Study the drawing (mm; zero at the part's minimum x, y, z) and answer. A direction names the side the tool comes from. Coordinates: 2 decimals unless noted, no trailing zeros. Loops run counter-clockwise (first coordinate to the right, second up) from the corner with the lowest first, then second, coordinate; pieces in that order, holes last. Notation, with made-up numbers: (86, 57.25) - (118, 57.25) arc R28 cw to (118, 91.25) - close; hole circle Ø1 at (45, 24). An arc over 180 degrees is marked (long way). Use one line per item in the form item = value.
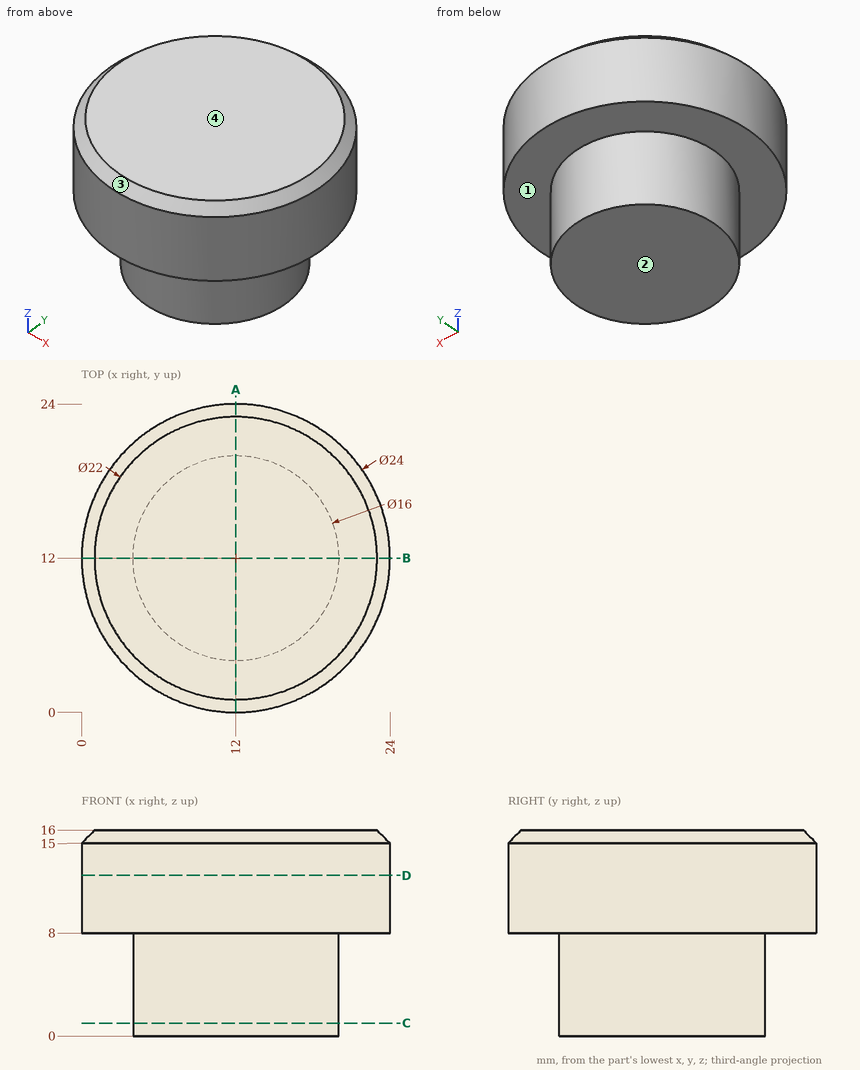
Item 1: The part is cut by section C-C on z = 1. Give the vertices of the cut face in (x, y).
Results below:
outline = circle Ø16 at (12, 12)
Item 2: For a pull along X with two mould halves and no side action, classify the marked faces 3 and 4 as +X half, -X half, draft (parallel to the pull), parting line (faces both ways), or undercut.
Results below:
face_3 = parting line
face_4 = draft
Item 3: The part is cut by section D-D on z = 12.5. Give the vertices of the cut face in (x, y), plus the area to 3 significant figures.
Results below:
outline = circle Ø24 at (12, 12)
area = 452 mm²
Item 4: Each of these flat-tipped pins is pushed along its axis until it touches: P1, Ø2, axis at x = 21, y = 16, coming from the -Z side; P2, Ø1.5, axis at y = 3.5, z = 14, coming from the -X side; P3, Ø2, axis at x = 20, z = 14, coming from the -Y side; P4, Ø5, axis at x = 15, y = 16.5, coming from the -Z side. Where does it stop, or does it pass through?
Results below:
P1 = 8
P2 = 2.84
P3 = 2.25
P4 = 0
Item 5: The part is cut by section A-A on x = 12. Give the vertices of the cut face in (y, z).
Results below:
outline = (0, 8) - (4, 8) - (4, 0) - (20, 0) - (20, 8) - (24, 8) - (24, 15) - (23, 16) - (1, 16) - (0, 15) - close
Item 6: Which of the six approach directions +Z, -Z, +X, -X, +Y, -Y give full straight-line access (tool end or side, diameter ignored) to the marked faces 1 and 2?
Results below:
face_1 = -Z
face_2 = -Z, +X, -X, +Y, -Y
Item 7: Find the intervals of material crossed by L1, parallel to Z at x = 6.25, y = 5.75; L2, parallel to Y at x = 12, z = 12.75; L3, parallel to Y at x = 19.5, z = 12.5, in increasing order.
Results below:
L1 = 8 to 16
L2 = 0 to 24
L3 = 2.63 to 21.37
